The listing builds one solid part. Answer for the finished solid, in the listing's coordinates (mm). Face numbers are marked on the shaded views. A direction names the side the tool comes from. Give positions to 0.01 mm unless a question says otherwise; leave off trailing zeros. Loops run counter-clockwise (first coordinate to the right, second up) from the corner with the lowest first, then second, coordinate; pieces in that order, holes last.
Item 1: The mould has two halves that part along Y. Classify the marked faces 1, 2 and 3: pulls with the +Y half, pulls with the -Y half, needs draft (parallel to the pull), parting line crosses it, or undercut.
Item 2: Section C-C, the plane z = -2.25 is taken. Give the vertices of the cut face in (x, y).
Item 3: Section A-A, the plane z = 1.5 is taken. Give the vertices of the cut face in (x, y), and give its area (3 significant figures).
Item 4: Consider line 1 along Z through (x, y) = (-0.5, -0.4); line 2 along Z through (x, y) = (1, -0.9); line 3 along X through (y, z) = (0.35, 1.5). Determine where each line is inside the solid, lowest interval first.
Item 5: Each of these flat-tipped pins is pushed along its axis until it touches: pin 1 Ø1.2 at (x, y) = (0, 0.5) entering from +Z; pin 2 Ø2 at (x, z) = (0.5, -2.5) entering from -Y; pin 3 Ø2 at (y, z) = (1.5, -1.5) entering from -X; pin 4 Ø2 at (y, z) = (-0.5, 1.5) entering from -X. Where does it stop, or does it pass through?
Item 6: A tool of negligible diameter and unlimited length cuts with its end or side. For the marked faces 4, 5 and 6, from which of +Z, -Z, +X, -X, +Y, -Y can it reach the whole face along a straight path? Write none if from no direction.
Solid Edge part; units mm, degrees
sketch "Sketch1" plane through (0, 0, 0) normal (0, 0, 1) x (1, 0, 0)
  circle A0 centre (0, 0) radius 2.25
extrude "Protrusion1" add sketch "Sketch1" along normal blind 2.5
sketch "Sketch2" plane through (0, 0, 2.5) normal (0, 0, 1) x (0, 1, 0)
  line L0 (0, 1.1547) -> (1, 0.5774)
  line L1 (1, 0.5774) -> (1, -0.5774)
  line L2 (1, -0.5774) -> (0, -1.1547)
  line L3 (0, -1.1547) -> (-1, -0.5774)
  line L4 (-1, -0.5774) -> (-1, 0.5774)
  line L5 (-1, 0.5774) -> (0, 1.1547)
extrude "Cutout1" cut sketch "Sketch2" against normal blind 1.1
fillet "Round1" radius 0.25 1 edges at (-2.25, 0, 2.5)
sketch "Sketch3" plane through (0, 0, 0) normal (1, 0, 0) x (0, 1, 0)
  line L0 (-0.974, -8) -> (0, -8)
  line L1 (-1.25, -7.724) -> (-0.974, -8)
  line L2 (-1.25, -1.35) -> (-1.25, -7.724)
  line L3 (-0.974, -1.35) -> (-1.25, -1.35)
  line L4 (-0.974, -1.34) -> (-0.974, -1.35)
  line L5 (-1.25, -1.34) -> (-0.974, -1.34)
  line L6 (-1.25, -0.1) -> (-1.25, -1.34)
  arc A0 (-1.25, -0.1) -> (-1.35, 0) centre (-1.35, -0.1) ccw
revolve "RevolvedProtrusion1" add sketch "Sketch3" angle 360 about axis through (0, 0, -60.325) along (0, 0, 1) material side at (0, -0.487, -7.95)
cosmetic_thread "Thread1"
sketch "Sketch4" plane through (0, 0, 0) normal (0, -1, 0) x (1, 0, 0)
  line L0 (-1.15, 2.5) -> (0, 1.836)
revolve "RevolvedCutout1" cut sketch "Sketch4" angle 360 about axis through (0, 0, 57.15) along (0, 0, -1) material side at (-0.55, 0, 2.2113)
properties material "Stahl"
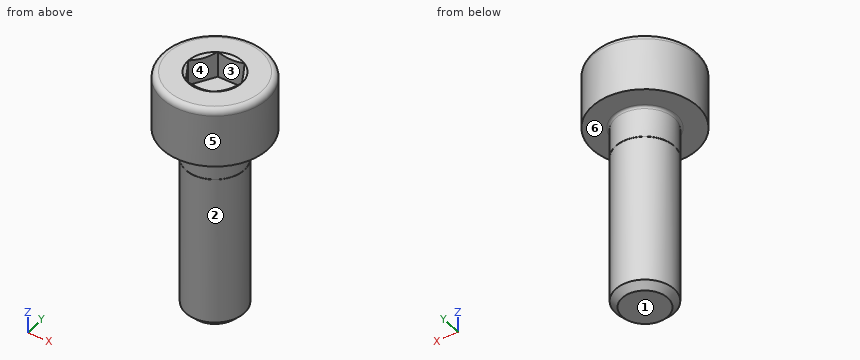
Worked answers:
1. face 1: needs draft
1. face 2: parting line crosses it
1. face 3: undercut
2. outline: circle Ø2.5 at (0, 0)
3. outline: circle Ø4.5 at (0, 0); hole (-1.15, 0) - (-0.58, -1) - (0.58, -1) - (1.15, 0) - (0.58, 1) - (-0.58, 1) - close
3. area: 12.4 mm2
4. line 1: z = -8 to 1.4
4. line 2: z = 0 to 2.5
4. line 3: x = -2.22 to -0.95, 0.95 to 2.22
5. pin 1: stops at z = 2.47
5. pin 2: stops at y = -1.25
5. pin 3: stops at x = -1.15
5. pin 4: stops at x = -2.25
6. face 4: +Z
6. face 5: +Z, -Z
6. face 6: -Z
